Geometry check sheet. Reference: the model listing, model coordinates, mm. Face numbers are marked on the shaded views. A direction names the side the tool comes from. Give positions to 0.01 mm unless a question says otherwise; leave off trailing zeros. Write each loop counter-clockwise with the first axis right and the second up, starting at its lowest first coordinate (ties: lowest second). Pieces come first, ordered by that corner, then holes. Notation, with made-up numbers: (11, 81.25) - (46, 81.25) arc R18 ccw to (46, 108.25) - close; hole circle Ø6 at (-14, 11). An arc over 180 degrees is marked (long way). One line per question, with ' | ' between items. Start each with the question number.
Q1. Gauge pin test, flat ends, axial feed: P1, Ø2, axis at x = 17.5, y = -7.5, coming from the -Z side; P2, Ø1.3, axis at y = -14.5, z = -0.5, coming from the -X side; P3, Ø1.5, axis at x = 56, y = -7, coming from the -Z side. Record the tip position at first contact, or that the pin passes through.
Q2. Set-up check for the marked faces 4, 5 and 6: record each of +Z, -Z, +X, -X, +Y, -Y from which the full face is reachable in a straight line by a thin tool's end or side.
Q3. Section check A-A on x = 47. Record the boundary of the cut face in (y, z), and give its area (3 significant figures).
Q4. Section check B-B on z = -43. Record the boundary of the cut face in (x, y), and give its area (3 significant figures).
Q5. Section check C-C on x = -27. Count the separate pieces of the cut face and the enclosed holes in it, and give its area (3 significant figures).
Q6. Thickness scan on L1, parallel to X at y = -7.5, z = 26; L2, parallel to Z at x = 58, y = -6; L3, parallel to Z at x = 42.5, y = -7. Record the ranges inside material, lowest first. Write a range as [from, to].
Q7. Release check for a two-part mould opening along X. For the marked faces 1, 2 and 3 record: +X half, -X half, draft (parallel to the pull), parting line (faces both ways), or undercut.
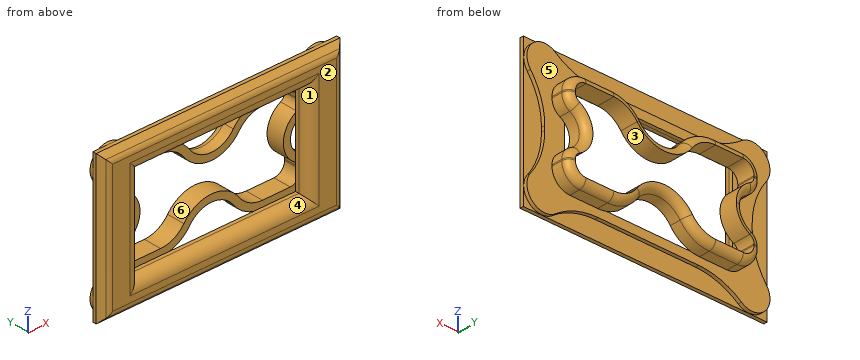
```python
from build123d import *

# Parameters (mm, degrees)
F0_W      = 137.6357078552
F0_H      = 68.2628676295
F1_DEPTH  = 12.7
F2_R      = 12.7
F5_DEPTH  = 25.4
F6_R      = 25.4
F8_DEPTH  = 25.4
F10_DEPTH = 25.4
F11_R     = 10.414
F12_R     = 5.08
F14_DEPTH = 25.4
F15_W     = 147.9870229959
F15_H     = 79.1546478868
F16_DEPTH = 2.54
F17_R     = 12.7
F18_DEPTH = 2.54
F19_R     = 50.8
F20_R     = 50.8
F21_R     = 50.8
F22_R     = 50.8
F23_W     = 173.9475429058
F23_H     = 104.9968674779
F24_DEPTH = 7.62
F25_SIZE  = 5.08
F26_R     = 5.08
F27_W     = 119.8056712747
F27_H     = 66.657833755
F28_DEPTH = 10.16
F29_R     = 7.62


with BuildPart() as f1:
    # F0 (on Front) → F1 (new body)
    with BuildSketch(Plane.XZ):
        Rectangle(F0_W, F0_H)
    extrude(amount=F1_DEPTH)

    # F2
    f2_edges = [f1.edges().sort_by_distance(p)[0] for p in [
        (-68.817854, -6.35, 34.131434),
        (68.817854, -6.35, 34.131434),
        (68.817854, -6.35, -34.131434),
        (-68.817854, -6.35, -34.131434),
    ]]
    fillet(f2_edges, radius=F2_R)

    # F4 (on face) → F5 (cut)
    with BuildSketch(Plane.XZ.offset(12.7)):
        with BuildLine():
            Line((-19.1200878216, -34.1314338148), (19.1200878216, -34.1314338148))
            ThreePointArc((19.1200878216, -34.1314338148), (0, -15.3615530935), (-19.1200878216, -34.1314338148))
        make_face()
        with BuildLine():
            ThreePointArc((-19.0234345987, 34.1314338148), (0, 15.3648180736), (19.0234345987, 34.1314338148))
            Line((19.0234345987, 34.1314338148), (-19.0234345987, 34.1314338148))
        make_face()
    extrude(amount=-F5_DEPTH, mode=Mode.SUBTRACT)

    # F6
    f6_edges = [f1.edges().sort_by_distance(p)[0] for p in [
        (-19.120088, -6.35, -34.131434),
        (19.120088, -6.35, -34.131434),
        (-19.023435, -6.35, 34.131434),
        (19.023435, -6.35, 34.131434),
    ]]
    fillet(f6_edges, radius=F6_R)

    # F3 (on face) → F8 (cut)
    with BuildSketch(Plane.XZ.offset(12.7)):
        with BuildLine():
            ThreePointArc((-68.8178539276, -12.7), (-59.8375978065, -8.9802561211), (-56.1178539276, 0))
            ThreePointArc((-56.1178539276, 0), (-59.8375978065, 8.9802561211), (-68.8178539276, 12.7))
            Line((-68.8178539276, 12.7), (-68.8178539276, -12.7))
        make_face()
    extrude(amount=-F8_DEPTH, mode=Mode.SUBTRACT)

    # F9 (on face) → F10 (cut)
    with BuildSketch(Plane.XZ.offset(12.7)):
        with BuildLine():
            Line((68.8178539276, -12.7031007157), (68.8178539276, 12.7031007157))
            ThreePointArc((68.8178539276, 12.7031007157), (56.2983967758, 0), (68.8178539276, -12.7031007157))
        make_face()
    extrude(amount=-F10_DEPTH, mode=Mode.SUBTRACT)

    # F11
    f11_edges = [f1.edges().sort_by_distance(p)[0] for p in [
        (-68.817854, -6.35, 12.7),
        (-68.817854, -6.35, -12.7),
        (68.817854, -6.35, -12.703101),
        (68.817854, -6.35, 12.703101),
    ]]
    fillet(f11_edges, radius=F11_R)

    # F12
    f12_edges = [f1.edges().sort_by_distance(p)[0] for p in [
        (68.817854, 0, 20.988545),
        (67.2969, 0, 15.126696),
        (65.09811, 0, 30.41169),
        (56.298397, 0, 0),
        (46.192012, 0, 34.131434),
        (67.2969, 0, -15.126696),
        (24.592779, 0, 31.290067),
        (68.817854, 0, -20.988545),
        (0, 0, 15.364818),
        (65.09811, 0, -30.41169),
        (-24.592779, 0, 31.290067),
        (46.21855, 0, -34.131434),
        (-46.192012, 0, 34.131434),
        (24.657717, 0, -31.296201),
        (-65.09811, 0, 30.41169),
        (0, 0, -15.361553),
        (-68.817854, 0, 21.033246),
        (-24.657717, 0, -31.296201),
        (-67.272735, 0, 15.176638),
        (-46.21855, 0, -34.131434),
        (-56.117854, 0, 0),
        (-65.09811, 0, -30.41169),
        (-67.272735, 0, -15.176638),
        (-68.817854, 0, -21.033246),
    ]]
    fillet(f12_edges, radius=F12_R)

    # F13 (on face) → F14 (cut)
    with BuildSketch(Plane(origin=(0, 0, 0), x_dir=(-1, 0, 0), z_dir=(0, 1, 0))):
        with BuildLine():
            ThreePointArc((-56.1178539276, 29.0514338148), (-61.5060076003, 26.8195874874), (-63.7378539276, 21.4314338148))
            Line((-63.7378539276, 21.4314338148), (-63.7378539276, 20.5456569949))
            ThreePointArc((-63.7378539276, 20.5456569949), (-62.9588285714, 17.7700918282), (-60.8493042485, 15.8052636854))
            ThreePointArc((-60.8493042485, 15.8052636854), (-51.2183967758, 0), (-60.8493042485, -15.8052636854))
            ThreePointArc((-60.8493042485, -15.8052636854), (-62.9588285714, -17.7700918282), (-63.7378539276, -20.5456569949))
            Line((-63.7378539276, -20.5456569949), (-63.7378539276, -21.4314338148))
            ThreePointArc((-63.7378539276, -21.4314338148), (-61.5060076003, -26.8195874874), (-56.1178539276, -29.0514338148))
            Line((-56.1178539276, -29.0514338148), (-36.3192469491, -29.0514338148))
            ThreePointArc((-36.3192469491, -29.0514338148), (-26.9900229374, -26.7832475558), (-19.7435172043, -20.4850538286))
            ThreePointArc((-19.7435172043, -20.4850538286), (0, -10.2815530935), (19.7435172043, -20.4850538286))
            ThreePointArc((19.7435172043, -20.4850538286), (26.9900229374, -26.7832475558), (36.3192469491, -29.0514338148))
            Line((36.3192469491, -29.0514338148), (56.1178539276, -29.0514338148))
            ThreePointArc((56.1178539276, -29.0514338148), (61.5060076003, -26.8195874874), (63.7378539276, -21.4314338148))
            Line((63.7378539276, -21.4314338148), (63.7378539276, -20.6350575478))
            ThreePointArc((63.7378539276, -20.6350575478), (62.9464516934, -17.8392818882), (60.8070846968, -15.8731211906))
            ThreePointArc((60.8070846968, -15.8731211906), (51.0378539276, 0), (60.8070846968, 15.8731211906))
            ThreePointArc((60.8070846968, 15.8731211906), (62.9464516934, 17.8392818882), (63.7378539276, 20.6350575478))
            Line((63.7378539276, 20.6350575478), (63.7378539276, 21.4314338148))
            ThreePointArc((63.7378539276, 21.4314338148), (61.5060076003, 26.8195874874), (56.1178539276, 29.0514338148))
            Line((56.1178539276, 29.0514338148), (36.2661707874, 29.0514338148))
            ThreePointArc((36.2661707874, 29.0514338148), (26.9274577492, 26.7783404414), (19.6780918294, 20.467618735))
            ThreePointArc((19.6780918294, 20.467618735), (0, 10.2848180736), (-19.6780918294, 20.467618735))
            ThreePointArc((-19.6780918294, 20.467618735), (-26.9274577492, 26.7783404414), (-36.2661707874, 29.0514338148))
            Line((-36.2661707874, 29.0514338148), (-56.1178539276, 29.0514338148))
        make_face()
    extrude(amount=-F14_DEPTH, mode=Mode.SUBTRACT)

    # F15 (on face) → F16 (join)
    with BuildSketch(Plane.XZ.offset(12.7)):
        Rectangle(F15_W, F15_H)
    extrude(amount=F16_DEPTH)

    # F17 (on face) → F18 (join)
    with BuildSketch(Plane.XZ.offset(15.24)):
        with Locations((-73.993511498, 39.5773239434)):
            Circle(F17_R)
        with Locations((73.993511498, 39.5773239434)):
            Circle(F17_R)
        with Locations((-73.993511498, -39.5773239434)):
            Circle(F17_R)
        with Locations((73.993511498, -39.5773239434)):
            Circle(F17_R)
    extrude(amount=-F18_DEPTH)

    # F19
    f19_edges = [f1.edges().sort_by_distance(p)[0] for p in [
        (61.293511, -13.97, 39.577324),
        (-61.293511, -13.97, 39.577324),
    ]]
    fillet(f19_edges, radius=F19_R)

    # F20
    f20_edges = [f1.edges().sort_by_distance(p)[0] for p in [
        (-73.993511, -13.97, 26.877324),
        (-61.293511, -13.97, -39.577324),
        (61.293511, -13.97, -39.577324),
    ]]
    fillet(f20_edges, radius=F20_R)

    # F21
    f21_edges = [f1.edges().sort_by_distance(p)[0] for p in [
        (-73.993511, -13.97, -26.877324),
    ]]
    fillet(f21_edges, radius=F21_R)

    # F22
    f22_edges = [f1.edges().sort_by_distance(p)[0] for p in [
        (73.993511, -13.97, -26.877324),
        (73.993511, -13.97, 26.877324),
    ]]
    fillet(f22_edges, radius=F22_R)

    # F23 (on face) → F24 (join)
    with BuildSketch(Plane.XZ.offset(15.24)):
        Rectangle(F23_W, F23_H)
        with BuildLine():
            ThreePointArc((84.153511498, -31.9573239434), (82.973767619, -48.5575800644), (66.373511498, -49.7373239434))
            ThreePointArc((66.373511498, -49.7373239434), (51.9578820116, -42.1842124024), (35.893511498, -39.5773239434))
            Line((35.893511498, -39.5773239434), (-35.893511498, -39.5773239434))
            ThreePointArc((-35.893511498, -39.5773239434), (-51.9578820116, -42.1842124024), (-66.373511498, -49.7373239434))
            ThreePointArc((-66.373511498, -49.7373239434), (-82.973767619, -48.5575800644), (-84.153511498, -31.9573239434))
            ThreePointArc((-84.153511498, -31.9573239434), (-76.600399957, -17.541694457), (-73.993511498, -1.4773239434))
            Line((-73.993511498, -1.4773239434), (-73.993511498, 1.4773239434))
            ThreePointArc((-73.993511498, 1.4773239434), (-76.600399957, 17.541694457), (-84.153511498, 31.9573239434))
            ThreePointArc((-84.153511498, 31.9573239434), (-82.973767619, 48.5575800644), (-66.373511498, 49.7373239434))
            ThreePointArc((-66.373511498, 49.7373239434), (-51.9578820116, 42.1842124024), (-35.893511498, 39.5773239434))
            Line((-35.893511498, 39.5773239434), (35.893511498, 39.5773239434))
            ThreePointArc((35.893511498, 39.5773239434), (51.9578820116, 42.1842124024), (66.373511498, 49.7373239434))
            ThreePointArc((66.373511498, 49.7373239434), (82.973767619, 48.5575800644), (84.153511498, 31.9573239434))
            ThreePointArc((84.153511498, 31.9573239434), (76.600399957, 17.541694457), (73.993511498, 1.4773239434))
            Line((73.993511498, 1.4773239434), (73.993511498, -1.4773239434))
            ThreePointArc((73.993511498, -1.4773239434), (76.600399957, -17.541694457), (84.153511498, -31.9573239434))
        make_face(mode=Mode.SUBTRACT)
        with BuildLine():
            ThreePointArc((35.893511498, -39.5773239434), (51.9578820116, -42.1842124024), (66.373511498, -49.7373239434))
            ThreePointArc((66.373511498, -49.7373239434), (82.973767619, -48.5575800644), (84.153511498, -31.9573239434))
            ThreePointArc((84.153511498, -31.9573239434), (76.600399957, -17.541694457), (73.993511498, -1.4773239434))
            Line((73.993511498, -1.4773239434), (73.993511498, 1.4773239434))
            ThreePointArc((73.993511498, 1.4773239434), (76.600399957, 17.541694457), (84.153511498, 31.9573239434))
            ThreePointArc((84.153511498, 31.9573239434), (82.973767619, 48.5575800644), (66.373511498, 49.7373239434))
            ThreePointArc((66.373511498, 49.7373239434), (51.9578820116, 42.1842124024), (35.893511498, 39.5773239434))
            Line((35.893511498, 39.5773239434), (-35.893511498, 39.5773239434))
            ThreePointArc((-35.893511498, 39.5773239434), (-51.9578820116, 42.1842124024), (-66.373511498, 49.7373239434))
            ThreePointArc((-66.373511498, 49.7373239434), (-82.973767619, 48.5575800644), (-84.153511498, 31.9573239434))
            ThreePointArc((-84.153511498, 31.9573239434), (-76.600399957, 17.541694457), (-73.993511498, 1.4773239434))
            Line((-73.993511498, 1.4773239434), (-73.993511498, -1.4773239434))
            ThreePointArc((-73.993511498, -1.4773239434), (-76.600399957, -17.541694457), (-84.153511498, -31.9573239434))
            ThreePointArc((-84.153511498, -31.9573239434), (-82.973767619, -48.5575800644), (-66.373511498, -49.7373239434))
            ThreePointArc((-66.373511498, -49.7373239434), (-51.9578820116, -42.1842124024), (-35.893511498, -39.5773239434))
            Line((-35.893511498, -39.5773239434), (35.893511498, -39.5773239434))
        make_face()
    extrude(amount=F24_DEPTH)

    # F25
    f25_edges = [f1.edges().sort_by_distance(p)[0] for p in [
        (0, -22.86, 52.498434),
        (-86.973771, -22.86, 0),
        (0, -22.86, -52.498434),
        (86.973771, -22.86, 0),
    ]]
    chamfer(f25_edges, length=F25_SIZE)

    # F26
    f26_edges = [f1.edges().sort_by_distance(p)[0] for p in [
        (-81.893771, -22.86, 0),
        (0, -22.86, -47.418434),
        (0, -22.86, 47.418434),
        (81.893771, -22.86, 0),
    ]]
    fillet(f26_edges, radius=F26_R)

    # F27 (on face) → F28 (cut)
    with BuildSketch(Plane.XZ.offset(22.86)):
        Rectangle(F27_W, F27_H)
    extrude(amount=-F28_DEPTH, mode=Mode.SUBTRACT)

    # F29
    f29_edges = [f1.edges().sort_by_distance(p)[0] for p in [
        (-79.789567, -22.86, 0),
        (0, -22.86, 45.314229),
        (0, -22.86, -45.314229),
        (79.789567, -22.86, 0),
        (0, -22.86, 33.328917),
        (-59.902836, -22.86, 0),
        (0, -22.86, -33.328917),
        (59.902836, -22.86, 0),
    ]]
    fillet(f29_edges, radius=F29_R)


solid = f1.part
```
Working result:
1) P1: stops at z = -26.83 | P2: stops at x = -73.99 | P3: stops at z = -34.13
2) face 4: -Y | face 5: +Y | face 6: +Y, -Y
3) outline: (-22.86, -45.31) arc R5.08 ccw to (-21.37, -48.91) - (-17.78, -52.5) - (-15.24, -52.5) - (-15.24, -40.81) - (-12.7, -40.81) - (-12.7, -34.13) - (-5.08, -34.13) arc R5.08 ccw to (0, -29.05) - (-12.7, -29.05) - (-12.7, -33.33) - (-15.24, -33.33) arc R7.62 ccw to (-22.86, -40.95) - close; (-22.86, 40.95) arc R7.62 ccw to (-15.24, 33.33) - (-12.7, 33.33) - (-12.7, 29.05) - (0, 29.05) arc R5.08 ccw to (-5.08, 34.13) - (-12.7, 34.13) - (-12.7, 40.81) - (-15.24, 40.81) - (-15.24, 52.5) - (-17.78, 52.5) - (-21.37, 48.91) arc R5.08 ccw to (-22.86, 45.31) - close | area: 396 mm2
4) outline: (-86.97, -17.78) - (-83.38, -21.37) arc R5.08 ccw to (-79.79, -22.86) - (79.79, -22.86) arc R5.08 ccw to (83.38, -21.37) - (86.97, -17.78) - (86.97, -15.24) - (86.22, -15.24) - (86.22, -12.7) - (54.22, -12.7) - (54.22, -15.24) - (-54.22, -15.24) - (-54.22, -12.7) - (-86.22, -12.7) - (-86.22, -15.24) - (-86.97, -15.24) - close | area: 1,460 mm2
5) separate pieces: 4 | enclosed holes: 0 | area: 401 mm2
6) L1: x = [-67.97, -62.22], [-25.56, -17.64], [17.64, 25.56], [62.22, 67.97] | L2: z = [-33.99, -28.82], [-13.97, -6.35], [6.35, 13.97], [28.82, 33.99] | L3: z = [-34.13, -29.05], [29.05, 34.13]
7) face 1: undercut | face 2: draft | face 3: undercut
